```python
from build123d import *

# Parameters (mm, degrees)
SKETCH1_W           = 104.14
SKETCH1_H           = 27.94
SKETCH1_R           = 3.175
BOSS_EXTRUDE1_DEPTH = 24.13
SKETCH2_W           = 41.91
SKETCH2_H           = 20.32
CUT_EXTRUDE1_DEPTH  = 16.51
CUT_EXTRUDE2_DEPTH  = 16.51
FILLET1_R           = 2.54


with BuildPart() as part:
    # Sketch1 → Boss-Extrude1 (new body)
    with BuildSketch(Plane(origin=(0, 0, 0), x_dir=(1, 0, 0), z_dir=(0, 1, 0))):
        Rectangle(SKETCH1_W, SKETCH1_H)
        with Locations(Location((40.005, 0, 0), (0, 0, 90))):
            Circle(SKETCH1_R, mode=Mode.SUBTRACT)
        with Locations(Location((-40.005, 0, 0), (0, 0, 90))):
            Circle(SKETCH1_R, mode=Mode.SUBTRACT)
    extrude(amount=BOSS_EXTRUDE1_DEPTH)

    # Sketch2 → Cut-Extrude1 (cut)
    with BuildSketch(Plane.XZ):
        with Locations((0, 3.81)):
            Rectangle(SKETCH2_W, SKETCH2_H)
    extrude(amount=-CUT_EXTRUDE1_DEPTH, mode=Mode.SUBTRACT)

    # Sketch4 → Cut-Extrude2 (cut)
    with BuildSketch(Plane(origin=(0, 24.13, 0), x_dir=(1, 0, 0), z_dir=(0, 1, 0))):
        Polygon((-52.07, -13.97), (-26.924, -13.97), (-20.066, 13.97), (-52.07, 13.97), align=None)
        Polygon((52.07, 13.97), (20.066, 13.97), (26.924, -13.97), (52.07, -13.97), align=None)
    extrude(amount=-CUT_EXTRUDE2_DEPTH, mode=Mode.SUBTRACT)

    # Fillet1
    fillet1_edges = [part.edges().sort_by_distance(p)[0] for p in [
        (-20.955, 8.255, -6.35),
        (0, 16.51, -6.35),
        (20.955, 8.255, -6.35),
        (52.07, 3.81, 13.97),
        (0, 24.13, 13.97),
        (-52.07, 3.81, 13.97),
        (-52.07, 3.81, -13.97),
        (0, 24.13, -13.97),
        (52.07, 3.81, -13.97),
        (-52.07, 7.62, 0),
        (-36.068, 7.62, -13.97),
        (-23.495, 7.62, 0),
        (-20.066, 15.875, -13.97),
        (-39.497, 7.62, 13.97),
        (-26.924, 15.875, 13.97),
        (-23.495, 24.13, 0),
        (52.07, 7.62, 0),
        (39.497, 7.62, 13.97),
        (23.495, 7.62, 0),
        (26.924, 15.875, 13.97),
        (36.068, 7.62, -13.97),
        (20.066, 15.875, -13.97),
        (23.495, 24.13, 0),
    ]]
    fillet(fillet1_edges, radius=FILLET1_R)


solid = part.part
```
CAD build for the part. Positions are in the model's coordinates, mm. A direction names the side the tool comes from. Coordinates: 2 decimals unless noted, no trailing zeros. Write each loop counter-clockwise with the first axis right and the second up, starting at its lowest first coordinate (ties: lowest second). Pieces come first, ordered by that corner, then holes. Notation, with made-up numbers: (54.5, 21.25) -> (77.5, 21.25) arc R25 cw to (77.5, 51.25) -> close; hole circle Ø9 at (11, 78). An arc over 180 degrees is marked (long way). Return JSON: item names as keys, results as strings. Group by question number.
Q1. Flat gauge pins, fed straight in: pin 1 (7 mm diameter, centred on x = -34.5, z = -5, fed in from +Y); pin 2 (4 mm diameter, centred on y = 7.5, z = 6, fed in from +X); pin 3 (1 mm diameter, centred on x = -9, z = -3.5, fed in from -Y); pin 4 (4 mm diameter, centred on x = 40.005, z = 0, fed in from -Y). Where does each tip first touch, or does it go through?
Q2. Cut at B-B, the plane x = -3. Give the cut face in (y, z), then the cut area to 3 significant figures.
Q3. Which spindle directions (+Z, -Z, +X, -X, +Y, -Y) get a long thin tool onto all of the face, cutting with end or side? Do faces 4 (the face through (36.2, 6.9, -13.2)), 5 (the face through (-19.623, 15.795, -13.443)), 6 (the face through (20.231, 8.371, -5.586)). Say none if no direction does.
Q4. Cut at C-C, the plane y = 18.25. Give the cut face in (x, z), then the cut area to 3 significant figures.
Q5. Drill centre lines: line 1 (X direction, y = 4.5, z = 0) (3 decimals); line 2 (X direction, y = 2.75, z = 10.5) (3 decimals); line 3 (Z direction, x = 7, y = 3.75). Where is each one in solid material? Low to high.
Q6. Pull direction X, two halves, no side cores. Call faces 1 (the face through (-20.191, 8.371, -5.626)), 2 (the face through (52.07, 3, 0)), 3 (the face through (-25.664, 15.795, 13.023)): released by +X, released by -X, zero draft, split by the parting line, or undercut.
Q7. Cut at A-A, the plane y = 3.25. Give the cut face in (x, z) (3 decimals), then the cut area to 3 significant figures.
Q8. Cut at D-D, the plane z = 0. State how many separate pieces and enclosed holes the cut face has, then the cut area to 3 significant figures.
Returned:
{
 "1": {"pin 1": "stops at y = 7.62", "pin 2": "stops at x = 52.04", "pin 3": "stops at y = 16.5", "pin 4": "passes through"},
 "2": {"outline": "(0, -13.97) -> (21.59, -13.97) arc R2.54 ccw to (24.13, -11.43) -> (24.13, 11.43) arc R2.54 ccw to (21.59, 13.97) -> (16.51, 13.97) -> (16.51, -3.81) arc R2.54 cw to (13.97, -6.35) -> (0, -6.35) -> close", "area": "337 mm2"},
 "3": {"face 4": "-Z, +X, +Y", "face 5": "-Z, -X, +Y", "face 6": "+Z, -Y"},
 "4": {"outline": "(-26.15, 10.82) -> (-20.54, -12.04) arc R2.54 ccw to (-18.07, -13.97) -> (18.07, -13.97) arc R2.54 ccw to (20.54, -12.04) -> (26.15, 10.82) arc R2.54 ccw to (23.69, 13.97) -> (-23.69, 13.97) arc R2.54 ccw to start", "area": "1,310 mm2"},
 "5": {"line 1": "x = -52.07 to -43.18, -36.83 to -20.955, 20.955 to 36.83, 43.18 to 52.07", "line 2": "x = -52.07 to -20.955, 20.955 to 52.07", "line 3": "z = -13.97 to -6.35"},
 "6": {"face 1": "undercut", "face 2": "released by +X", "face 3": "released by -X"},
 "7": {"outline": "(-52.07, -11.43) arc R2.54 ccw to (-49.53, -13.97) -> (49.53, -13.97) arc R2.54 ccw to (52.07, -11.43) -> (52.07, 11.43) arc R2.54 ccw to (49.53, 13.97) -> (20.955, 13.97) -> (20.955, -3.81) arc R2.54 cw to (18.415, -6.35) -> (-18.415, -6.35) arc R2.54 cw to (-20.955, -3.81) -> (-20.955, 13.97) -> (-49.53, 13.97) arc R2.54 ccw to (-52.07, 11.43) -> close; hole circle Ø6.35 at (-40.005, 0); hole circle Ø6.35 at (40.005, 0)", "area": "1,990 mm2"},
 "8": {"separate pieces": "3", "enclosed holes": "0", "area": "778 mm2"}
}
